from build123d import *

# Parameters (mm, degrees)
SKETCH1_W           = 30
SKETCH1_H           = 16
BOSS_EXTRUDE1_DEPTH = 10
BOSS_EXTRUDE2_DEPTH = 4
SKETCH3_R           = 1
CUT_EXTRUDE1_DEPTH  = 20


with BuildPart() as part:
    # Sketch1 → Boss-Extrude1 (new body)
    with BuildSketch(Plane(origin=(0, 0, 0), x_dir=(1, 0, 0), z_dir=(0, 1, 0))):
        Polygon((83.598365037, 72.861095688), (19.188679245, 4.528301887), (19.188679245, -3.471698113), (67.093699226, 33.50154619), (99.126439745, 58.224515545), align=None)
        Polygon((75.084307937, -20.878636135), (19.188679245, -3.471698113), (19.188679245, -11.471698113), (150.692912318, -66.106409411), (156.848103065, -46.341402143), align=None)
        with Locations((4.188679245, -3.471698113)):
            Rectangle(SKETCH1_W, SKETCH1_H)
        Polygon((67.093699226, 33.50154619), (19.188679245, -3.471698113), (75.084307937, -20.878636135), align=None)
    extrude(amount=BOSS_EXTRUDE1_DEPTH)

    # Sketch2 → Boss-Extrude2 (add)
    with BuildSketch(Plane(origin=(0, 10, 0), x_dir=(1, 0, 0), z_dir=(0, 1, 0))):
        with BuildLine():
            Line((-4.616424759, 0.799624641), (21.383575241, 0.799624641))
            ThreePointArc((21.383575241, 0.799624641), (25.477598736, -3.294398854), (21.383575241, -7.38842235))
            Line((21.383575241, -7.38842235), (-4.616424759, -7.38842235))
            ThreePointArc((-4.616424759, -7.38842235), (-8.710448255, -3.294398854), (-4.616424759, 0.799624641))
        make_face()
    extrude(amount=BOSS_EXTRUDE2_DEPTH)

    # Sketch3 → Cut-Extrude1 (cut)
    with BuildSketch(Plane(origin=(0, 14, 0), x_dir=(1, 0, 0), z_dir=(0, 1, 0))):
        with Locations(Location((-2.189535813, -3.38842235, 0), (0, 0, 270))):
            Circle(SKETCH3_R)
        with Locations(Location((7.810464187, -3.394168988, 0), (0, 0, 270))):
            Circle(SKETCH3_R)
    extrude(amount=-CUT_EXTRUDE1_DEPTH, mode=Mode.SUBTRACT)


solid = part.part
Input: part model. Units: mm. Frame: model coordinates. A direction names the side the tool comes from. Coordinates: 2 decimals unless noted, no trailing zeros. Order: outer loops, then holes, each group sorted by start corner. A loop starts at its lowest first (then second) coordinate and runs counter-clockwise, first axis right, second up. Notation, with made-up numbers: M 60,-35 L 107,-35 A27 ccw 107,-6 Z; hole C -17,67.25 d10. An arc over 180 degrees is marked long. Answer in a Markdown table with one row per item.
(1) Material intervals for line 1 (Z direction, x = 12, y = 5.5); line 2 (Z direction, x = 7, y = 13.25); line 3 (Y direction, x = 58, z = -19), sorted ascending. Write a range as [from, to].
Numbers:
| item | result |
|---|---|
| line 1 | z = [-4.53, 11.47] |
| line 2 | z = [-0.8, 2.81], [3.98, 7.39] |
| line 3 | y = [0, 10] |
(2) Section query B-B, the plane y = 1.75. Output: boundary loops of the cut face in (x, z).
Numbers:
| item | result |
|---|---|
| outline | M -10.81,-4.53 L 19.19,-4.53 L 83.6,-72.86 L 99.13,-58.22 L 67.09,-33.5 L 75.08,20.88 L 156.85,46.34 L 150.69,66.11 L 19.19,11.47 L -10.81,11.47 Z; hole C -2.19,3.39 d2; hole C 7.81,3.39 d2 |
(3) Section query C-C, the plane x = 71. Output: boundary loops of the cut face in (y, z).
Numbers:
| item | result |
|---|---|
| outline | M 0,-59.5 L 10,-59.5 L 10,-36.52 L 0,-36.52 Z; M 0,-6.92 L 10,-6.92 L 10,33 L 0,33 Z |
(4) Contact query for flat-ended pins moving along their axis: pin 1 Ø3 at (x, y) = (11, 12) entering from +Z; pin 2 Ø3 at (x, y) = (66.5, 9.5) entering from +Z; pin 3 Ø5 at (x, y) = (109.5, 11.5) entering from -Z. Output: stop coordinate, or through.
Numbers:
| item | result |
|---|---|
| pin 1 | stops at z = 7.39 |
| pin 2 | stops at z = 31.75 |
| pin 3 | stops at z = 30.97 |
(5) Draft query along Z for faces 1 (the flat face through (66, 0, 1)), 2 (the flat face through (91.47, 4.93, -65.44)), 3 (the flat face through (116.54, 4.93, 33.79)), 4 (the flat face through (82.9, 4.9, -45.7)). Return one class per face: pulls with the +Z half, pulls with the -Z half, needs draft (parallel to the pull), parting line crosses it, or undercut.
Numbers:
| item | result |
|---|---|
| face 1 | needs draft |
| face 2 | pulls with the -Z half |
| face 3 | undercut |
| face 4 | undercut |
(6) Access query for faces 5 (the flat face through (4, 5, 11.472)), 6 (the cylindrical face through (-8.71, 11.97, 3.38)), 7 (the flat face through (8, 12, -0.8)), 8 (the flat face through (71.145, 4.93, -5.931)), 9 (the flat face through (4, 5, -4.528)). Directions: +Z, -Z, +X, -X, +Y, -Y. A direction counts if a zero-diameter tool reaches every point of the face in a straight line with its end or side. Return the directions, or none.
Numbers:
| item | result |
|---|---|
| face 5 | +Z, -X, +Y, -Y |
| face 6 | -X, +Y |
| face 7 | -Z, +X, -X, +Y |
| face 8 | +X, +Y, -Y |
| face 9 | -Z, -X, +Y, -Y |
(7) Section query A-A, the plane x = 2. Output: boundary loops of the cut face in (y, z), plus the area to 3 significant figures.
Numbers:
| item | result |
|---|---|
| outline | M 0,-4.53 L 10,-4.53 L 10,-0.8 L 14,-0.8 L 14,7.39 L 10,7.39 L 10,11.47 L 0,11.47 Z |
| area | 193 mm^2 |
(8) Section query D-D, the plane z = 41.5. Output: boundary loops of the cut face in (x, y).
Numbers:
| item | result |
|---|---|
| outline | M 91.47,0 L 141.3,0 L 141.3,10 L 91.47,10 Z |
